Read the model definition and answer for the solid it produces. Units are mm, in the model's axes. A direction names the side the tool comes from. Give positions to 0.01 mm unless a question says otherwise; leave off trailing zeros. Order: outer loops, then holes, each group sorted by start corner. A loop starts at its lowest first (then second) coordinate and runs counter-clockwise, first axis right, second up. Notation, with made-up numbers: (83, 67.25) - (121, 67.25) arc R17 ccw to (121, 76.25) - close; hole circle Ø5 at (-9, -30.75). An arc over 180 degrees is marked (long way). Write item = value, one per line.
```python
from build123d import *

# Parameters (mm, degrees)
SKETCH1_R           = 1.5
BOSS_EXTRUDE1_DEPTH = 3
SKETCH2_R           = 2.5
BOSS_EXTRUDE2_DEPTH = 0.001


with BuildPart() as part:
    # Sketch1 → Boss-Extrude1 (new body)
    with BuildSketch(Plane(origin=(0, 0, 0), x_dir=(1, 0, 0), z_dir=(0, 1, 0))):
        with BuildLine():
            Line((1.470120334, 47.615099655), (39.019477518, 26.493586162))
            ThreePointArc((39.019477518, 26.493586162), (40, 26.236737235), (40.980522482, 26.493586162))
            Line((40.980522482, 26.493586162), (78.529879666, 47.615099655))
            ThreePointArc((78.529879666, 47.615099655), (82.614620243, 46.470972803), (81.471825115, 42.385859447))
            Line((81.471825115, 42.385859447), (49.218121455, 24.243151073))
            ThreePointArc((49.218121455, 24.243151073), (48.198643937, 22.5), (49.218121455, 20.756848927))
            Line((49.218121455, 20.756848927), (81.471825115, 2.614140553))
            ThreePointArc((81.471825115, 2.614140553), (82.614620243, -1.470972803), (78.529879666, -2.615099655))
            Line((78.529879666, -2.615099655), (40.980522482, 18.506413838))
            ThreePointArc((40.980522482, 18.506413838), (40, 18.763262765), (39.019477518, 18.506413838))
            Line((39.019477518, 18.506413838), (1.470120334, -2.615099655))
            ThreePointArc((1.470120334, -2.615099655), (-2.614620243, -1.470972803), (-1.471825115, 2.614140553))
            Line((-1.471825115, 2.614140553), (30.781878545, 20.756848927))
            ThreePointArc((30.781878545, 20.756848927), (31.801356063, 22.5), (30.781878545, 24.243151073))
            Line((30.781878545, 24.243151073), (-1.471825115, 42.385859447))
            ThreePointArc((-1.471825115, 42.385859447), (-2.614620243, 46.470972803), (1.470120334, 47.615099655))
        make_face()
        with Locations(Location((0, 45, 0), (0, 0, 270))):
            Circle(SKETCH1_R, mode=Mode.SUBTRACT)
        with Locations(Location((80, 45, 0), (0, 0, 270))):
            Circle(SKETCH1_R, mode=Mode.SUBTRACT)
        with Locations(Location((80, 0, 0), (0, 0, 270))):
            Circle(SKETCH1_R, mode=Mode.SUBTRACT)
        with Locations(Location((0, 0, 0), (0, 0, 270))):
            Circle(SKETCH1_R, mode=Mode.SUBTRACT)
    extrude(amount=BOSS_EXTRUDE1_DEPTH)

    # Sketch2 → Boss-Extrude2 (add)
    with BuildSketch(Plane(origin=(0, 3, 0), x_dir=(1, 0, 0), z_dir=(0, 1, 0))):
        with Locations(Location((39.97951418, 22.909712694, 0), (0, 0, 270))):
            Circle(SKETCH2_R)
    extrude(amount=BOSS_EXTRUDE2_DEPTH)


solid = part.part
```
1. Section D-D (z = -7) is taken. Determine the outline of the cut face in (x, y), and give its area (3 significant figures).
Recorded:
outline = (6.33, 0) - (18.56, 0) - (18.56, 3) - (6.33, 3) - close; (61.44, 0) - (73.67, 0) - (73.67, 3) - (61.44, 3) - close
area = 73.4 mm^2
2. Flat-ended cylindrical pins translate along their axes: pin 1 (1 mm diameter, centred on y = 0.5, z = -35.5, fed in from +X); pin 2 (4 mm diameter, centred on x = 0, z = 0, fed in from +Y). Find the tip coordinate at first contact, or state that the pin passes through.
Recorded:
pin_1 = 70.12
pin_2 = 3
3. For faces 5 (the face through (-2.6, 1.5, 1.5)), 6 (the face through (43, 3, -23)), 7 (the face through (60.018, 1.479, -7.798)), 8 (the face through (65.12, 1.48, -11.81)), 9 (the face through (14.88, 1.48, -33.19)), determine the directions among +Z, -Z, +X, -X, +Y, -Y from which every point of the face is accessible in a straight line to the end or side of a thin tool.
Recorded:
face_5 = +Y, -Y
face_6 = +Z, -Z, +X, -X, +Y
face_7 = +Z, +Y, -Y
face_8 = +X, +Y, -Y
face_9 = -X, +Y, -Y
4. Section B-B (z = -45) is taken. Determine the outline of the cut face in (x, y), and give its area (3 significant figures).
Recorded:
outline = (-3, 0) - (-1.5, 0) - (-1.5, 3) - (-3, 3) - close; (1.5, 0) - (6.12, 0) - (6.12, 3) - (1.5, 3) - close; (73.88, 0) - (78.5, 0) - (78.5, 3) - (73.88, 3) - close; (81.5, 0) - (83, 0) - (83, 3) - (81.5, 3) - close
area = 36.7 mm^2
5. Determine the mould class of faces 1 (the face through (31.8, 1.5, -22.5)), 2 (the face through (20.508, 1.479, -8.094)), 3 (the face through (-2.65, 1.48, -46.41)), 4 (the face through (40, 3.001, -23)) for opening direction Z: +Z half, -Z half, draft (parallel to the pull), parting line (faces both ways), or undercut.
Recorded:
face_1 = undercut
face_2 = +Z half
face_3 = undercut
face_4 = draft
6. Section A-A (y = 1.2) is taken. Determine the outline of the cut face in (x, z), and give its area (3 significant figures).
Recorded:
outline = (-1.47, -42.39) arc R3 ccw to (1.47, -47.62) - (39.02, -26.49) arc R2 cw to (40.98, -26.49) - (78.53, -47.62) arc R3 ccw to (81.47, -42.39) - (49.22, -24.24) arc R2 cw to (49.22, -20.76) - (81.47, -2.61) arc R3 ccw to (78.53, 2.62) - (40.98, -18.51) arc R2 cw to (39.02, -18.51) - (1.47, 2.62) arc R3 ccw to (-1.47, -2.61) - (30.78, -20.76) arc R2 cw to (30.78, -24.24) - close; hole circle Ø3 at (0, -45); hole circle Ø3 at (0, 0); hole circle Ø3 at (80, -45); hole circle Ø3 at (80, 0)
area = 1,090 mm^2
7. Section C-C (x = 80) is taken. Determine the outline of the cut face in (y, z).
Recorded:
outline = (0, -48) - (3, -48) - (3, -46.5) - (0, -46.5) - close; (0, -43.5) - (3, -43.5) - (3, -41.56) - (0, -41.56) - close; (0, -3.44) - (3, -3.44) - (3, -1.5) - (0, -1.5) - close; (0, 1.5) - (3, 1.5) - (3, 3) - (0, 3) - close
8. Straight lines are drawn through the part: L1, parallel to X at y = 1.65, z = 0; L2, parallel to Z at x = 80, y = 2.15; L3, parallel to Z at x = 58, y = 0.3. For each, find the intervals that lie inside material, in ascending order. Write a range as [from, to].
Recorded:
L1 = [-3, -1.5], [1.5, 6.12], [73.88, 78.5], [81.5, 83]
L2 = [-48, -46.5], [-43.5, -41.56], [-3.44, -1.5], [1.5, 3]
L3 = [-36.07, -29.18], [-15.82, -8.93]
